Autodesk Inventor part; units mm, degrees
ref_plane "YZ Plane" through (0, 0, 0) normal (1, 0, 0) x (0, 1, 0)
ref_plane "XZ Plane" through (0, 0, 0) normal (0, 1, 0) x (-1, 0, 0)
ref_plane "XY Plane" through (0, 0, 0) normal (0, 0, 1) x (1, 0, 0)
sketch "Sketch1" plane through (0, 0, 0) normal (1, 0, 0) x (0, 1, 0)
  line L0 (0, 0) -> (0, -19.05)
  line L1 (0, -19.05) -> (12.7, -19.05)
  line L2 (12.7, -19.05) -> (12.7, -15.875)
  line L3 (12.7, -15.875) -> (3.175, -15.875)
  line L4 (3.175, -15.875) -> (3.175, 0)
  line L5 (3.175, 0) -> (0, 0)
  dimension "d0" = 3.175
  dimension "d1" = 12.7
  dimension "d4" = 3.175
  dimension "d5" = 19.05
extrude "Extrusion1" add sketch "Sketch1" along normal blind 12.7
sketch "Sketch3" plane through (0, 3.175, 0) normal (0, 1, 0) x (1, 0, 0)
  line L0 (0, 15.875) -> (0, 0)
  line L1 (0, 0) -> (12.7, 0)
  line L2 (12.7, 15.875) -> (12.7, 0)
  line L3 (0, 15.875) -> (12.7, 15.875)
  point P0 (0, 0)
  point P1 (6.35, 7.9375)
hole "Hole2" at (6.35, 3.175, -7.9375) direction (0, -1, 0) diameter 10.16 depth 2.032
sketch "Sketch4" plane through (0, 0, -19.05) normal (0, 0, -1) x (-1, 0, 0)
  line L0 (0, 12.7) -> (-12.7, 12.7)
  line L1 (0, 0) -> (-12.7, 0)
  line L2 (-8.89, 12.7) -> (-3.81, 12.7)
  line L3 (-3.81, 12.7) -> (-3.81, 0)
  line L4 (-3.81, 0) -> (-8.89, 0)
  line L5 (-8.89, 0) -> (-8.89, 12.7)
  line L6 (0, 0) -> (0, 12.7)
  line L7 (0, 12.7) -> (-12.7, 12.7)
  line L8 (-12.7, 0) -> (-12.7, 12.7)
  line L9 (0, 0) -> (-12.7, 0)
  dimension "d22" = 5.08
  dimension "d23" = 12.7
  dimension "d24" = 3.81
extrude "Extrusion2" add sketch "Sketch4" along normal blind 1.5875 contours L3 L1 L5 L0
sketch "Sketch5" plane through (0, 3.175, -15.875) normal (0, 0, 1) x (1, 0, 0)
  line L0 (0, 9.525) -> (0, 0)
  line L1 (0, 0) -> (12.7, 0)
  line L2 (12.7, 9.525) -> (12.7, 0)
  line L3 (0, 9.525) -> (12.7, 9.525)
  point P0 (0, -3.175)
  point P1 (6.3842, 4.8389)
hole "Hole3" at (6.3842, 8.0139, -15.875) direction (0, 0, -1) diameter 3.81 end through all counterbore diameter 6.35 counterbore depth 2.54
equation "\"d4\" = d0"
equation "\"d24\" = -0.5 * d22 + 0.5 * d23"
properties part number "spring tab for on arm"
Check sheet for the modelled part. Datum: model origin and axes. Units: mm. A direction names the side the tool comes from. Round coordinates to 2 decimals unless told otherwise and drop trailing zeros. Write each loop counter-clockwise with the first axis right and the second up, starting at its lowest first coordinate (ties: lowest second). Pieces come first, ordered by that corner, then holes. Notation, with made-up numbers: (89.5, 73.25) -> (122.5, 73.25) arc R26 ccw to (122.5, 102.25) -> close; hole circle Ø3 at (78.25, 65.25). An arc over 180 degrees is marked (long way). Answer as CSV lines item,"result". Start each with the question number.
1) Material ranges on line 1 (X direction, y = 2.75, z = -7.75); line 2 (Z direction, x = 6.35, y = 2.1); line 3 (Z direction, x = 10.75, y = 6.5) (3 decimals), recorded low to high. Write a range as from..to.
2) Section check C-C on z = -12. Enter the section's corners in (x, y) (3 decimals), and give its area (3 significant figures).
3) Go/stop test with flat-tipped pins: P1, Ø4, axis at y = 4.5, z = -14.5, coming from the -X side; P2, Ø3, axis at x = 11, y = 7, coming from the -Z side; P3, Ø6, axis at x = 6.35, z = -7.94, coming from the +Y side; P4, Ø6, axis at x = 6.38, y = 8.01, coming from the +Z side (3 decimals). Record where each tip stops, or that it passes through.
4) Section check A-A on x = 7. Enter the section's corners in (y, z) (1 decimal), and give its area (3 significant figures).
5) Release check for a two-part mould opening along X. For faces 5 (the flat face through (6, 1.143, -8)), 6 (the flat face through (2, 6, -19.05)), 7 (the flat face through (0, 3, -12)), 8 (the flat face through (8.89, 6, -20)) record: pulls with the +X half, pulls with the -X half, needs draft (parallel to the pull), parting line crosses it, or undercut.
6) Tool access check on faces 1 (the flat face through (11, 6, -19.05)), 2 (the flat face through (6.3, 5.9, -18.415)), 3 (the cylindrical face through (10.857, 2.145, -5.593)), 4 (the flat face through (8, 5, -15.875)). Record the directions out of +Z, -Z, +X, -X, +Y, -Y that give a thin tool (end or side, any length) a straight path to the whole face; none if there is none.
Found:
1,line 1,"x = 0..1.27, 11.43..12.7"
1,line 2,"z = -20.64..-13.02, -2.86..0"
1,line 3,"z = -19.05..-15.875"
2,outline,"(0, 0) -> (12.7, 0) -> (12.7, 3.175) -> (9.4, 3.175) -> (9.4, 1.143) -> (3.3, 1.143) -> (3.3, 3.175) -> (0, 3.175) -> close"
2,area,"27.9 mm^2"
3,P1,"stops at x = 0"
3,P2,"stops at z = -19.05"
3,P3,"stops at y = 1.14"
3,P4,"stops at z = -18.415"
4,outline,"(0, -20.6) -> (6.2, -20.6) -> (6.2, -18.4) -> (4.9, -18.4) -> (4.9, -15.9) -> (3.2, -15.9) -> (3.2, -13) -> (1.1, -13) -> (1.1, -2.9) -> (3.2, -2.9) -> (3.2, 0) -> (0, 0) -> close; (9.8, -20.6) -> (12.7, -20.6) -> (12.7, -15.9) -> (11.1, -15.9) -> (11.1, -18.4) -> (9.8, -18.4) -> close"
4,area,"66.6 mm^2"
5,face 5,"undercut"
5,face 6,"needs draft"
5,face 7,"pulls with the -X half"
5,face 8,"pulls with the +X half"
6,face 1,"-Z, +X, +Y, -Y"
6,face 2,"+Z"
6,face 3,"+Y"
6,face 4,"+Z, +X, -X, +Y"
